from build123d import *

# Parameters (mm, degrees)
BOSS_EXTRUDE1_DEPTH = 1.5
FILLET1_R           = 2


with BuildPart() as part:
    # Sketch1 → Boss-Extrude1 (new body)
    with BuildSketch(Plane.XY):
        with BuildLine():
            ThreePointArc((2.4, 4.5), (0, 15.475179423), (-2.4, 4.5))
            Line((-2.4, 4.5), (-2.4, 0))
            Line((-2.4, 0), (-5.5, 0))
            Line((-5.5, 0), (-5.5, 3.787942032))
            ThreePointArc((-5.5, 3.787942032), (0, 20.475179423), (5.5, 3.787942032))
            Line((5.5, 3.787942032), (5.5, 0))
            Line((5.5, 0), (2.4, 0))
            Line((2.4, 0), (2.4, 4.5))
        make_face()
    extrude(amount=BOSS_EXTRUDE1_DEPTH)

    # Fillet1
    fillet1_edges = [part.edges().sort_by_distance(p)[0] for p in [
        (-5.5, 3.787942032, 0.75),
        (5.5, 3.787942032, 0.75),
    ]]
    fillet(fillet1_edges, radius=FILLET1_R)


solid = part.part
Could you check a few things on this model? Use its own coordinates, in mm. A direction names the side the tool comes from. Coordinates: 2 decimals unless noted, no trailing zeros. Write each loop counter-clockwise with the first axis right and the second up, starting at its lowest first coordinate (ties: lowest second). Pieces come first, ordered by that corner, then holes. Notation, with made-up numbers: (11.5, 39.25) - (65.5, 39.25) arc R30 cw to (65.5, 61.25) - close; hole circle Ø10 at (38, 12.5). An arc over 180 degrees is marked (long way). Put each result on its own line as item: value. Start each with the question number.
Q1. Which directions (+Z, -Z, +X, -X, +Y, -Y) give clear straight access to the entire face, cutting with the end or side of a thin tool? Please do faces 4 (the flat face through (-5.5, 1, 1)), 5 (the flat face through (2.4, 2, 1)), 6 (the flat face through (5.5, 1, 1)).
Q2. I want a section at B-B on z = 1.1. Write out the boundary of the cut face in (x, y), plus the area to 3 significant figures.
Q3. I want a section at D-D on x = 0. Write out the boundary of the cut face in (y, z).
Q4. Thinking about a two-plate mould opening in Y: for faces 1 (the flat face through (-4, 15, 1.5)), 2 (the cylindrical face through (-0.31, 20.47, 0.74)), 3 (the cylindrical face through (0.22, 15.47, 0.74)), which applies, pulls with the +Y half, pulls with the -Y half, needs draft (parallel to the pull), parting line crosses it, or undercut?
Q5. Please list where these lines run through material, in increasing order: L1, parallel to X at y = 2.5, z = 0.2; L2, parallel to Y at x = 0, z = 0.55; L3, parallel to X at y = 5, z = 0.4.
Q6. I want a section at C-C on x = -4. Write out the boundary of the cut face in (y, z), plus the area to 3 significant figures.
Q7. I want a section at A-A on y = 11. Write out the boundary of the cut face in (x, z), plus the area to 3 significant figures.
Checks:
1. face 4: +Z, -Z, -X, -Y
1. face 5: +Z, -Z, -Y
1. face 6: +Z, -Z, +X, -Y
2. outline: (-6.17, 4.33) arc R2 cw to (-5.5, 2.84) - (-5.5, 0) - (-2.4, 0) - (-2.4, 4.5) arc R5.75 cw (long way) to (2.4, 4.5) - (2.4, 0) - (5.5, 0) - (5.5, 2.84) arc R2 cw to (6.17, 4.33) arc R9.25 ccw (long way) to start
2. area: 173 mm²
3. outline: (15.48, 0) - (20.48, 0) - (20.48, 1.5) - (15.48, 1.5) - close
4. face 1: needs draft
4. face 2: parting line crosses it
4. face 3: undercut
5. L1: -5.5 to -2.4, 2.4 to 5.5
5. L2: 15.48 to 20.48
5. L3: -6.84 to -3.28, 3.28 to 6.84
6. outline: (0, 0) - (5.59, 0) - (5.59, 1.5) - (0, 1.5) - close; (13.86, 0) - (19.57, 0) - (19.57, 1.5) - (13.86, 1.5) - close
6. area: 17.0 mm²
7. outline: (-9.25, 0) - (-5.61, 0) - (-5.61, 1.5) - (-9.25, 1.5) - close; (5.61, 0) - (9.25, 0) - (9.25, 1.5) - (5.61, 1.5) - close
7. area: 10.9 mm²
